CAD build for the part. Positions are in the model's coordinates, mm. A direction names the side the tool comes from. Coordinates: 2 decimals unless noted, no trailing zeros. Loops run counter-clockwise (first coordinate to the right, second up) from the corner with the lowest first, then second, coordinate; pieces in that order, holes last. Notation, with made-up numbers: (-21, -9) -> (-3, -9) arc R11 cw to (-3, -2) -> close; hole circle Ø9 at (19, 85.5). An arc over 180 degrees is marked (long way). Answer as a JSON object with one key per item and string values. Group by question number.
from build123d import *

# Parameters (mm, degrees)
F1_DEPTH = 25
F3_DEPTH = 53.001
F6_DEPTH = 15
F8_DEPTH = 20.8


with BuildPart() as f1:
    # F0 (on Top) → F1 (new body)
    with BuildSketch(Plane.XY):
        with BuildLine():
            Line((23.5, 35), (-23.5, 35))
            ThreePointArc((-23.5, 35), (-25.62132, 34.12132), (-26.5, 32))
            Line((-26.5, 32), (-26.5, -32))
            ThreePointArc((-26.5, -32), (-25.62132, -34.12132), (-23.5, -35))
            Line((-23.5, -35), (23.5, -35))
            ThreePointArc((23.5, -35), (25.62132, -34.12132), (26.5, -32))
            Line((26.5, -32), (26.5, 32))
            ThreePointArc((26.5, 32), (25.62132, 34.12132), (23.5, 35))
        make_face()
    extrude(amount=F1_DEPTH)

    # F2 (on face) → F3 (cut, through all)
    with BuildSketch(Plane.YZ.offset(26.5)):
        Polygon((-35, 25), (-35, 0), (35, 16.160773), (35, 25), align=None)
    extrude(amount=-F3_DEPTH, mode=Mode.SUBTRACT)

    # F5 (on offset) → F6 (cut)
    with BuildSketch(Plane.XY.offset(25)):
        with BuildLine():
            Line((2.849753, 13.3125), (6.411945, 24.140625))
            ThreePointArc((6.411945, 24.140625), (0, 33), (-6.411945, 24.140625))
            Line((-6.411945, 24.140625), (-2.849753, 13.3125))
            ThreePointArc((-2.849753, 13.3125), (0, 11.25), (2.849753, 13.3125))
        make_face()
        with BuildLine():
            Line((19.849753, 13.3125), (23.411945, 24.140625))
            ThreePointArc((23.411945, 24.140625), (17, 33), (10.588055, 24.140625))
            Line((10.588055, 24.140625), (14.150247, 13.3125))
            ThreePointArc((14.150247, 13.3125), (17, 11.25), (19.849753, 13.3125))
        make_face()
        with BuildLine():
            ThreePointArc((-19.849753, 13.3125), (-17, 11.25), (-14.150247, 13.3125))
            Line((-14.150247, 13.3125), (-10.588055, 24.140625))
            ThreePointArc((-10.588055, 24.140625), (-17, 33), (-23.411945, 24.140625))
            Line((-23.411945, 24.140625), (-19.849753, 13.3125))
        make_face()
    extrude(amount=-F6_DEPTH, mode=Mode.SUBTRACT)

    # F7 (on offset) → F8 (cut)
    with BuildSketch(Plane.XY.offset(25)):
        with BuildLine():
            Line((10.588055, -0.859375), (14.150247, -11.6875))
            ThreePointArc((14.150247, -11.6875), (17, -13.75), (19.849753, -11.6875))
            Line((19.849753, -11.6875), (23.411945, -0.859375))
            ThreePointArc((23.411945, -0.859375), (17, 8), (10.588055, -0.859375))
        make_face()
        with BuildLine():
            ThreePointArc((-2.849753, -11.6875), (0, -13.75), (2.849753, -11.6875))
            Line((2.849753, -11.6875), (6.411945, -0.859375))
            ThreePointArc((6.411945, -0.859375), (0, 8), (-6.411945, -0.859375))
            Line((-6.411945, -0.859375), (-2.849753, -11.6875))
        make_face()
        with BuildLine():
            ThreePointArc((-19.849753, -11.6875), (-17, -13.75), (-14.150247, -11.6875))
            Line((-14.150247, -11.6875), (-10.588055, -0.859375))
            ThreePointArc((-10.588055, -0.859375), (-17, 8), (-23.411945, -0.859375))
            Line((-23.411945, -0.859375), (-19.849753, -11.6875))
        make_face()
    extrude(amount=-F8_DEPTH, mode=Mode.SUBTRACT)


solid = f1.part
Item 1: 3-axis set-ups, long thin cutter, end or side, ignore diameter. For faces 1 (the flat face through (17, -3, 4.2)), 2 (the cylindrical face through (25.64, 34.1, 7.97)): which of +Z, -Z, +X, -X, +Y, -Y reach the whole face in a straight line?
Item 2: Band-saw the part on A-A, the plane x = -15.5. List the corners of the cut face in (y, z), and give its area (3 significant figures).
Item 3: Band-saw the part on D-D, the plane x = 2. List the corners of the cut face in (y, z).
Item 4: Band-saw the part on B-B, the plane y = -8. List the corners of the cut face in (x, z).
Item 5: Band-saw the part on C-C, the plane z = 12. List the corners of the cut face in (x, y).
Item 6: Flat gauge pins, fed straight in: P1, Ø5, axis at x = 20, y = -12, coming from the +Z side; P2, Ø4, axis at x = -16, y = 1, coming from the +Z side; P3, Ø15, axis at x = 1, y = 26.5, coming from the +Z side. Where does each tip first touch, or does it go through?
Item 7: Pull direction Y, two halves, no side cores. Call faces 3 (the flat face through (0, -3, 4.2)), 4 (the flat face through (0, 35, 8)), 5 (the cylindrical face through (26.205, -33.298, 0.188)): +Y half, -Y half, draft (parallel to the pull), parting line (faces both ways), or undercut.
Item 8: Drill centre lines: L1, parallel to X at y = 1.25, z = 7.75; L2, parallel to X at y = 19, z = 10.5; L3, parallel to Z at x = 0, y = 18.5. Where is each one in solid material? Low to high.
Reply:
{
 "1": {"face 1": "+Z", "face 2": "+Z, -Z, +X, +Y"},
 "2": {"outline": "(-35, 0) -> (35, 0) -> (35, 16.16) -> (32.83, 15.66) -> (32.83, 10) -> (11.65, 10) -> (11.65, 10.77) -> (7.83, 9.89) -> (7.83, 4.2) -> (-13.35, 4.2) -> (-13.35, 5) -> close", "area": "429 mm²"},
 "3": {"outline": "(-35, 0) -> (35, 0) -> (35, 16.16) -> (32.7, 15.63) -> (32.7, 10) -> (12.01, 10) -> (12.01, 10.85) -> (7.7, 9.86) -> (7.7, 4.2) -> (-12.99, 4.2) -> (-12.99, 5.08) -> close"},
 "4": {"outline": "(-26.5, 0) -> (26.5, 0) -> (26.5, 6.23) -> (21.06, 6.23) -> (21.06, 4.2) -> (12.94, 4.2) -> (12.94, 6.23) -> (4.06, 6.23) -> (4.06, 4.2) -> (-4.06, 4.2) -> (-4.06, 6.23) -> (-12.94, 6.23) -> (-12.94, 4.2) -> (-21.06, 4.2) -> (-21.06, 6.23) -> (-26.5, 6.23) -> close"},
 "5": {"outline": "(-26.5, 16.98) -> (-21.06, 16.98) -> (-23.41, 24.14) arc R6.75 cw (long way) to (-10.59, 24.14) -> (-12.94, 16.98) -> (-4.06, 16.98) -> (-6.41, 24.14) arc R6.75 cw (long way) to (6.41, 24.14) -> (4.06, 16.98) -> (12.94, 16.98) -> (10.59, 24.14) arc R6.75 cw (long way) to (23.41, 24.14) -> (21.06, 16.98) -> (26.5, 16.98) -> (26.5, 32) arc R3 ccw to (23.5, 35) -> (-23.5, 35) arc R3 ccw to (-26.5, 32) -> close"},
 "6": {"P1": "z = 5.87", "P2": "z = 4.2", "P3": "z = 15.93"},
 "7": {"face 3": "undercut", "face 4": "+Y half", "face 5": "-Y half"},
 "8": {"L1": "-26.5 to -23.75, -10.25 to -6.75, 6.75 to 10.25, 23.75 to 26.5", "L2": "-26.5 to -21.72, -12.28 to -4.72, 4.72 to 12.28, 21.72 to 26.5", "L3": "0 to 10"}
}
